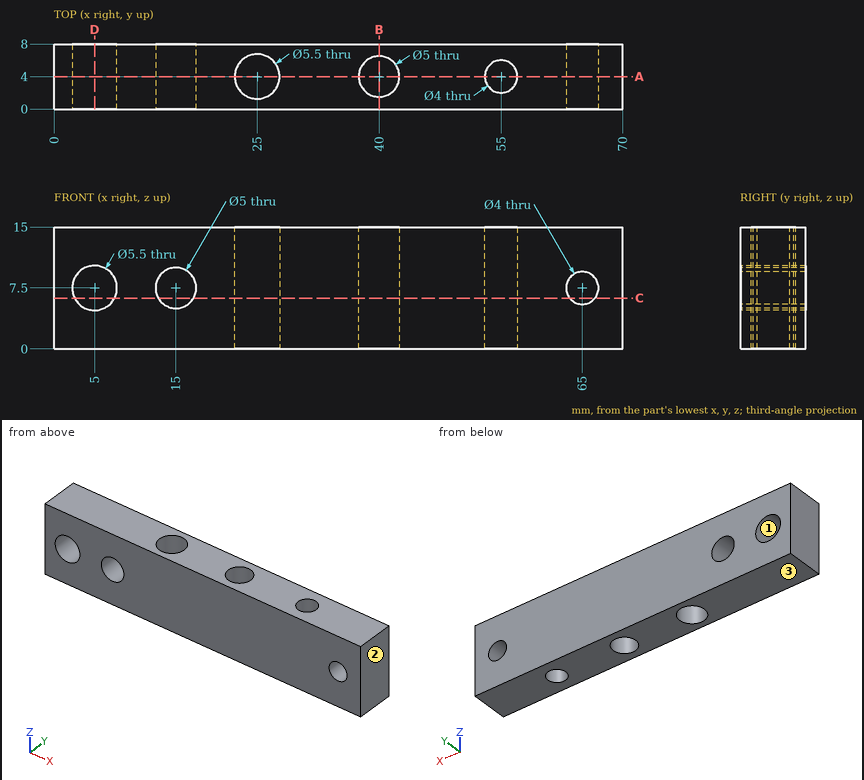
Input: dimensioned drawing with shaded views. Units: mm. Origin: part minimum x, y, z. Give positions to 0.01 mm unless a question says otherwise; leave off trailing zeros. Write each loop counter-clockwise with the first axis right and the second up, starting at its lowest first coordinate (ties: lowest second). Pieces come first, ordered by that corner, then holes.
Q1. Section D-D, the plane x = 5. Output: boundary loops of the cut face in (y, z).
Q2. Section B-B, the plane x = 40. Output: boundary loops of the cut face in (y, z), plus the area to 3 significant figures.
Q3. Material intervals for probe 1 along X at (y, z) = (4, 10.75); probe 2 along X at (y, z) = (3, 14.75); probe 3 along Z at (x, y) = (15, 6.25), sorted ascending.
Q4. Section A-A, the plane y = 4. Output: boundary loops of the cut face in (x, z).
Q5. Section C-C, the plane z = 6.25. Output: boundary loops of the cut face in (x, y).
Q6. Pull-direction query (Z, two-part tool) for the marked faces 1, 2 and 3; classes: pulls with the +Z half, pulls with the -Z half, needs draft (parallel to the pull), parting line crosses it, or undercut.
Q7. First-contact query: P1, Ø3.5, axis at x = 25, y = 4, coming from the -Z side. Flat tip, straight axial feed; report the tip coordinate or a pass-through.
Filled in:
1. outline: (0, 0) - (8, 0) - (8, 4.75) - (0, 4.75) - close; (0, 10.25) - (8, 10.25) - (8, 15) - (0, 15) - close
2. outline: (0, 0) - (1.5, 0) - (1.5, 15) - (0, 15) - close; (6.5, 0) - (8, 0) - (8, 15) - (6.5, 15) - close
2. area: 45.0 mm2
3. probe 1: x = 0 to 22.25, 27.75 to 37.5, 42.5 to 53, 57 to 70
3. probe 2: x = 0 to 22.44, 27.56 to 37.71, 42.29 to 53.27, 56.73 to 70
3. probe 3: z = 0 to 5, 10 to 15
4. outline: (0, 0) - (22.25, 0) - (22.25, 15) - (0, 15) - close; (27.75, 0) - (37.5, 0) - (37.5, 15) - (27.75, 15) - close; (42.5, 0) - (53, 0) - (53, 15) - (42.5, 15) - close; (57, 0) - (70, 0) - (70, 15) - (57, 15) - close; hole circle Ø5.5 at (5, 7.5); hole circle Ø5 at (15, 7.5); hole circle Ø4 at (65, 7.5)
5. outline: (0, 0) - (2.55, 0) - (2.55, 8) - (0, 8) - close; (7.45, 0) - (12.83, 0) - (12.83, 8) - (7.45, 8) - close; (17.17, 0) - (63.44, 0) - (63.44, 8) - (17.17, 8) - close; (66.56, 0) - (70, 0) - (70, 8) - (66.56, 8) - close; hole circle Ø5.5 at (25, 4); hole circle Ø5 at (40, 4); hole circle Ø4 at (55, 4)
6. face 1: undercut
6. face 2: needs draft
6. face 3: pulls with the -Z half
7. P1: passes through
